Check sheet for the drawn part. Datum: minimum x, y, z corner. Units: mm. A direction names the side the tool comes from. Coordinates: 2 decimals unless noted, no trailing zeros. Order: outer loops, then holes, each group sorted by start corner. A loop starts at its lowest first (then second) coordinate and runs counter-clockwise, first axis right, second up.
1. Thickness scan on line 1 (X direction, y = 1, z = 9.3); line 2 (Z direction, x = 28.75, y = 1.5); line 3 (Z direction, x = 21.25, y = 0.95). Record the ranges inside material, lowest first.
2. Cross-section at C-C (z = 5.75). Enter the section's corners in (x, y), then the cut area to 3 significant figures.
3. Set-up check for the marked faces 1 and 2: record each of +Z, -Z, +X, -X, +Y, -Y from which the full face is reachable in a straight line by a thin tool's end or side.
4. Cross-section at D-D (z = 13.25). Enter the section's corners in (x, y).
5. Cross-section at B-B (x = 28.75). Enter the section's corners in (y, z), then the cut area to 3 significant figures.
6. Cross-section at A-A (y = 11). Enter the section's corners in (x, z).
7. Gauge pin test, flat ends, axial feed: pin 1 Ø1 at (x, z) = (3.5, 14) entering from +Y; pin 2 Ø1.9 at (y, z) = (11, 14.25) entering from -X. Record the tip position at first contact, or that the pin passes through.
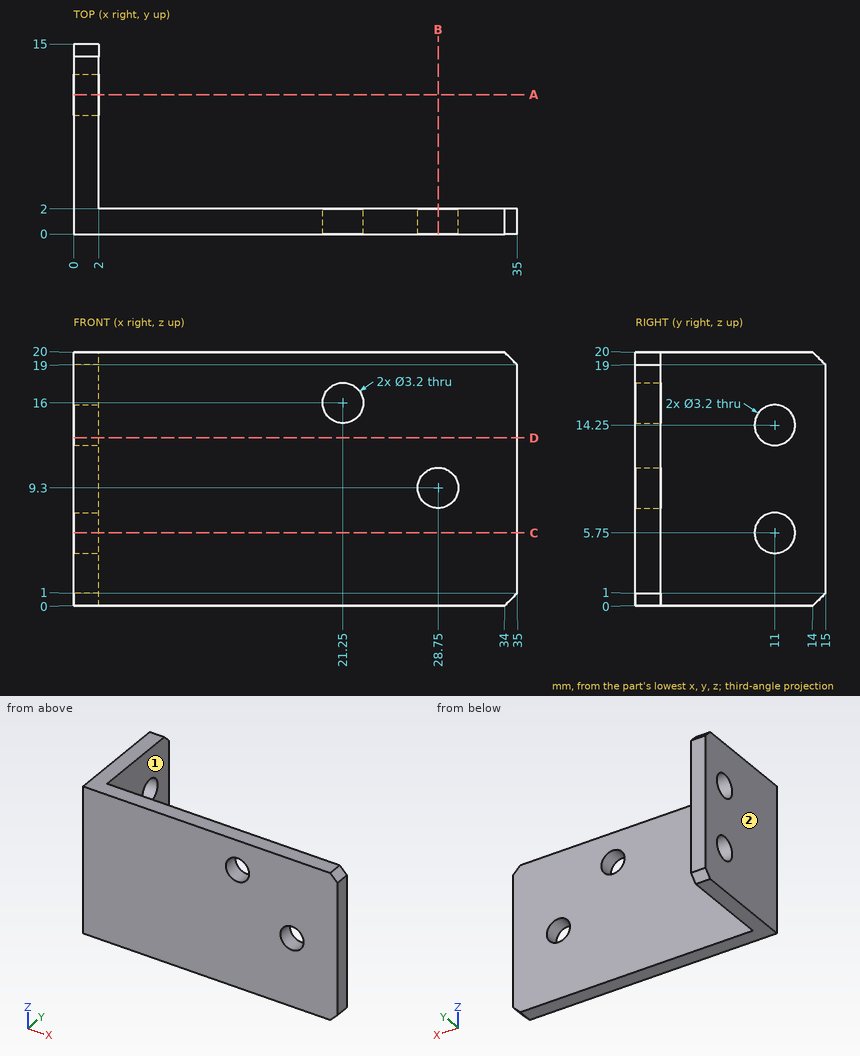
Data:
1. line 1: x = 0 to 27.15, 30.35 to 35
1. line 2: z = 0 to 7.7, 10.9 to 20
1. line 3: z = 0 to 14.4, 17.6 to 20
2. outline: (0, 0) - (35, 0) - (35, 2) - (2, 2) - (2, 9.4) - (0, 9.4) - close; (0, 12.6) - (2, 12.6) - (2, 15) - (0, 15) - close
2. area: 89.6 mm2
3. face 1: +Z, -Z, +X, +Y
3. face 2: +Z, -Z, -X, +Y, -Y
4. outline: (0, 0) - (35, 0) - (35, 2) - (2, 2) - (2, 9.75) - (0, 9.75) - close; (0, 12.25) - (2, 12.25) - (2, 15) - (0, 15) - close
5. outline: (0, 0) - (2, 0) - (2, 7.7) - (0, 7.7) - close; (0, 10.9) - (2, 10.9) - (2, 20) - (0, 20) - close
5. area: 33.6 mm2
6. outline: (0, 0) - (2, 0) - (2, 4.15) - (0, 4.15) - close; (0, 7.35) - (2, 7.35) - (2, 12.65) - (0, 12.65) - close; (0, 15.85) - (2, 15.85) - (2, 20) - (0, 20) - close
7. pin 1: stops at y = 2
7. pin 2: passes through
